Source: CAD feature listing. Evaluate the final solid. Frame: model axes, mm. Face numbers are marked on the shaded views. A direction names the side the tool comes from. Give positions to 0.01 mm unless a question says otherwise; leave off trailing zeros. Write each loop counter-clockwise with the first axis right and the second up, starting at its lowest first coordinate (ties: lowest second). Pieces come first, ordered by that corner, then holes.
```python
from build123d import *

# Parameters (mm, degrees)
F1_DEPTH = 25


with BuildPart() as f1:
    # F0 (on Front) → F1 (new body)
    with BuildSketch(Plane.XZ):
        with BuildLine():
            Line((-30, 140), (-40, 140))
            Line((-40, 140), (-40, 120))
            ThreePointArc((-40, 120), (-54.644661, 84.644661), (-90, 70))
            ThreePointArc((-90, 70), (-146.568542, 46.568542), (-170, -10))
            ThreePointArc((-170, -10), (-169.362376, -20.080343), (-167.459667, -30))
            Line((-167.459667, -30), (-110, -30))
            Line((-110, -30), (-110, -10))
            ThreePointArc((-110, -10), (-104.142136, 4.142136), (-90, 10))
            Line((-90, 10), (-58.284271, 10))
            ThreePointArc((-58.284271, 10), (-50.630603, 8.477591), (-44.142136, 4.142136))
            Line((-44.142136, 4.142136), (-21.213203, -18.786797))
            ThreePointArc((-21.213203, -18.786797), (0, -27.573593), (21.213203, -18.786797))
            Line((21.213203, -18.786797), (44.142136, 4.142136))
            ThreePointArc((44.142136, 4.142136), (50.630603, 8.477591), (58.284271, 10))
            Line((58.284271, 10), (140, 10))
            ThreePointArc((140, 10), (147.071068, 7.071068), (150, 0))
            Line((150, 0), (170, 0))
            Line((170, 0), (170, 80))
            Line((170, 80), (150, 80))
            ThreePointArc((150, 80), (147.071068, 72.928932), (140, 70))
            Line((140, 70), (90, 70))
            ThreePointArc((90, 70), (54.644661, 84.644661), (40, 120))
            Line((40, 120), (40, 140))
            Line((40, 140), (30, 140))
            Line((30, 140), (-30, 140))
        make_face()
        Polygon((-30, 160), (-30, 140), (30, 140), (30, 160), (10, 160), (-10, 160), align=None)
        with BuildLine():
            Line((-10, 202.679492), (-10, 160))
            Line((-10, 160), (10, 160))
            Line((10, 160), (10, 202.679492))
            ThreePointArc((10, 202.679492), (16.568043, 208.797324), (19.79899, 217.171573))
            ThreePointArc((19.79899, 217.171573), (20, 220), (19.79899, 222.828427))
            ThreePointArc((19.79899, 222.828427), (0, 240), (-19.79899, 222.828427))
            ThreePointArc((-19.79899, 222.828427), (-20, 220), (-19.79899, 217.171573))
            ThreePointArc((-19.79899, 217.171573), (-16.568043, 208.797324), (-10, 202.679492))
        make_face()
        with BuildLine():
            ThreePointArc((19.79899, 222.828427), (20, 220), (19.79899, 217.171573))
            Line((19.79899, 217.171573), (70, 210))
            Line((70, 210), (70, 230))
            Line((70, 230), (19.79899, 222.828427))
        make_face()
        with BuildLine():
            Line((-70, 210), (-19.79899, 217.171573))
            ThreePointArc((-19.79899, 217.171573), (-20, 220), (-19.79899, 222.828427))
            Line((-19.79899, 222.828427), (-70, 230))
            Line((-70, 230), (-70, 210))
        make_face()
    extrude(amount=F1_DEPTH)


solid = f1.part
```
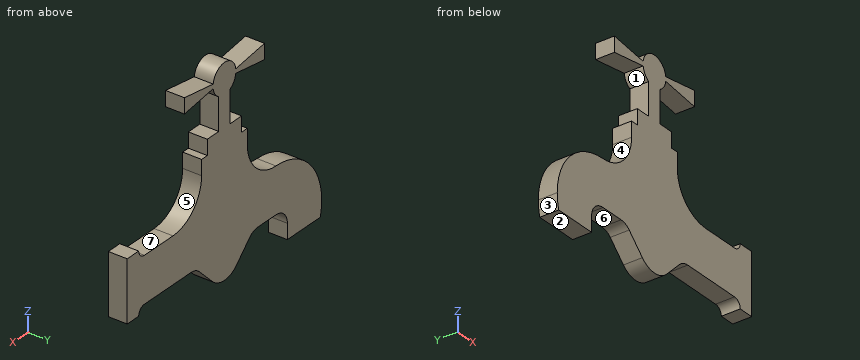
1. Line query: L1, parallel to X at y = -11, z = 123.5; L2, parallel to Z at x = 141, y = -19.5; L3, parallel to X at y = -22.25, z = -7. Output: solid intervals per line, ascending.
2. Cut plane C-C, the plane z = 34.5. Return the cut outline in (x, y), then the cut area to 3 significant figures.
3. Mould query, pull axis X, two halves, no side actions, for the marked faces 1, 2 and 3. Classes: +X half, -X half, draft (parallel to the pull), parting line (faces both ways), or undercut.
4. Cut plane D-D, the plane x = 103. Return the cut outline in (y, z).
5. Cut plane A-A, the plane x = -16. Return the cut outline in (y, z).
6. Contact query for flat-ended pins moving along their axis: P1, Ø7.5, axis at x = 117, y = -13.5, coming from the +Z side; P2, Ø10, axis at x = -2.5, y = -18, coming from the -Z side; P3, Ø6, axis at y = -14, z = 129, coming from the -X side; P4, Ø8, axis at x = 67, z = 48, coming from the +Y side. Output: stop coordinate, or through.
7. Access query for the marked faces 4, 5, 6 and 7. Directions: +Z, -Z, +X, -X, +Y, -Y. A direction counts if a zero-diameter tool reaches every point of the face in a straight line with its end or side. Return the directions, or none.
8. Cut plane B-B, the plane x = 53. Return the cut outline in (y, z).
Response values:
1. L1: x = -40 to 40
1. L2: z = 9.95 to 70.05
1. L3: x = -169.94 to -109.77, -33 to 33
2. outline: (-156.48, -25) - (170, -25) - (170, 0) - (-156.48, 0) - close
2. area: 8,160 mm2
3. face 1: undercut
3. face 2: draft
3. face 3: -X half
4. outline: (-25, 10) - (0, 10) - (0, 70) - (-25, 70) - close
5. outline: (-25, -22.95) - (0, -22.95) - (0, 160) - (-25, 160) - close; (-25, 208) - (0, 208) - (0, 232) - (-25, 232) - close
6. P1: stops at z = 70
6. P2: stops at z = -27.57
6. P3: stops at x = -40
6. P4: stops at y = 0
7. face 4: -X, +Y, -Y
7. face 5: +Y, -Y
7. face 6: -Z, +Y, -Y
7. face 7: +Z, +Y, -Y
8. outline: (-25, 9.29) - (0, 9.29) - (0, 86.37) - (-25, 86.37) - close; (-25, 212.43) - (0, 212.43) - (0, 227.57) - (-25, 227.57) - close
